Answer from the drawing. Dimensions are ordinates in mm from the lowest x, y and z of the part. A direction names the side the tool comes from. Coordinates: 2 decimals unless noted, no trailing zeros. Write each loop counter-clockwise with the first axis right and the second up, starting at its lowest first coordinate (ties: lowest second). Pieces come first, ordered by that corner, then holes.
(1) Given pin 1 (0.9 mm diameter, centred on x = 37.5, z = 26, fed in from -Y); pin 2 (7 mm diameter, centred on x = 6, z = 23, fed in from -Y), each flat-ended and moving along its own axis, determine where each tip first touches the part or whether it passes through.
(2) Straight lines are drawn through the part: line 1 along Z through (x, y) = (37, 3.5) (1 decimal); line 2 along Z through (x, y) = (17, 6) (1 decimal); line 3 along Z through (x, y) = (4, 6) (1 decimal). For each, find the intervals that lie inside material, in ascending order.
(3) The part is cut by section B-B, the plane x = 17. Determine the outline of the cut face in (y, z) (1 decimal).
(4) The part is cut by section A-A, the plane y = 3. State how many separate pieces and enclosed holes the cut face has, and give its area (3 significant figures).
(5) Determine the mould class of the marked faces 1, 2, 3 and 4 for opening direction X: pulls with the +X half, pulls with the -X half, needs draft (parallel to the pull), parting line crosses it, or undercut.
(6) The part is cut by section C-C, the plane x = 6. Determine the outline of the cut face in (y, z) (1 decimal).
(7) Which of the six approach directions +Z, -Z, +X, -X, +Y, -Y give full straight-line access (tool end or side, diameter ignored) to the marked faces 5 and 6?
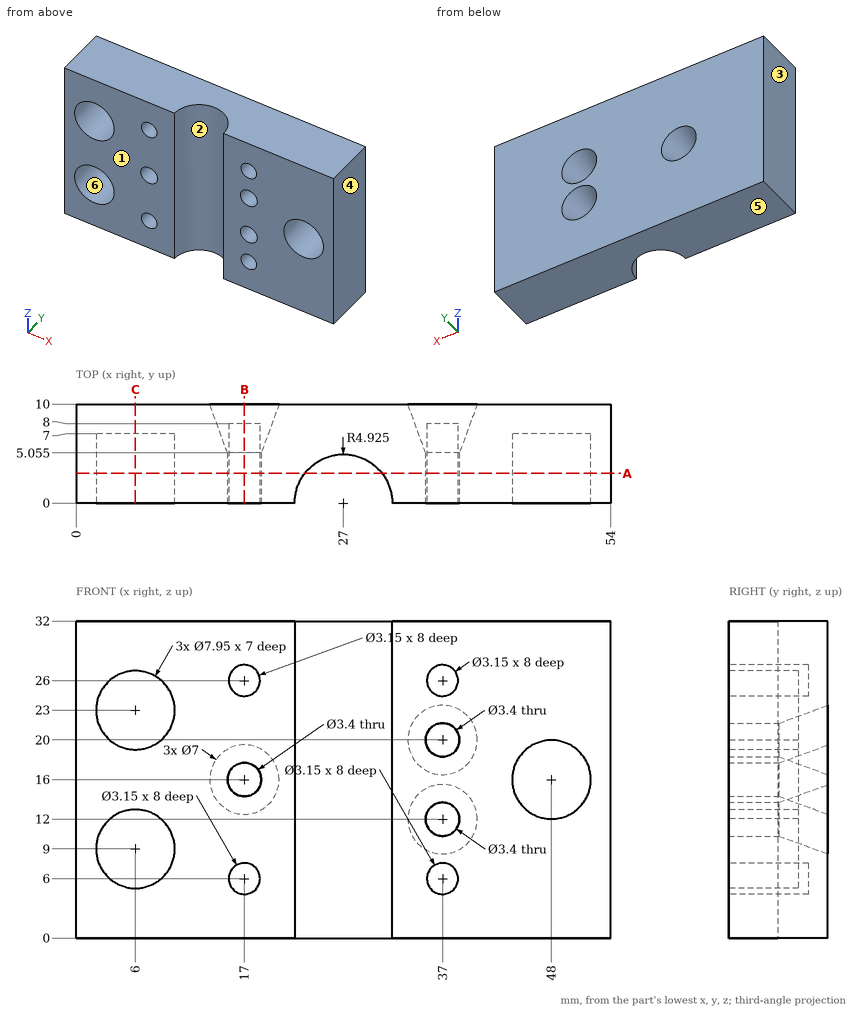
Computed:
1. pin 1: stops at y = 8
1. pin 2: stops at y = 7
2. line 1: z = 0 to 4.4, 7.6 to 10.3, 13.7 to 18.3, 21.7 to 24.4, 27.6 to 32
2. line 2: z = 0 to 4.4, 7.6 to 14, 18 to 24.4, 27.6 to 32
2. line 3: z = 0 to 5.6, 12.4 to 19.6, 26.4 to 32
3. outline: (0, 0) - (10, 0) - (10, 12.5) - (5.1, 14.3) - (0, 14.3) - (0, 7.6) - (8, 7.6) - (8, 4.4) - (0, 4.4) - close; (0, 17.7) - (5.1, 17.7) - (10, 19.5) - (10, 32) - (0, 32) - (0, 27.6) - (8, 27.6) - (8, 24.4) - (0, 24.4) - close
4. separate pieces: 2
4. enclosed holes: 10
4. area: 1,270 mm2
5. face 1: needs draft
5. face 2: undercut
5. face 3: pulls with the -X half
5. face 4: pulls with the +X half
6. outline: (0, 0) - (10, 0) - (10, 32) - (0, 32) - (0, 27) - (7, 27) - (7, 19) - (0, 19) - (0, 13) - (7, 13) - (7, 5) - (0, 5) - close
7. face 5: -Z, +X, -X, +Y, -Y
7. face 6: -Y
